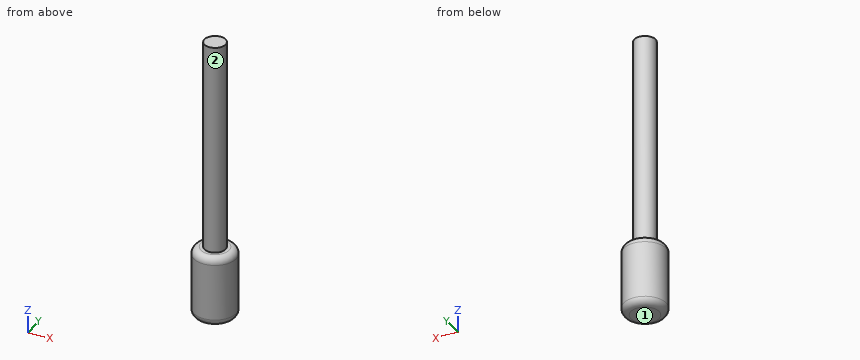
```python
from build123d import *

# Parameters (mm, degrees)
F0_R     = 15
F1_DEPTH = 50
F2_R     = 5
F3_R     = 7.5
F4_DEPTH = 150


with BuildPart() as f1:
    # F0 (on Top) → F1 (new body)
    with BuildSketch(Plane.XY):
        Circle(F0_R)
    extrude(amount=F1_DEPTH)

    # F2
    f2_edges = [f1.edges().sort_by_distance(p)[0] for p in [
        (-15, 0, 50),
        (-15, 0, 0),
    ]]
    fillet(f2_edges, radius=F2_R)

    # F3 (on face) → F4 (join)
    with BuildSketch(Plane.XY.offset(50)):
        Circle(F3_R)
    extrude(amount=F4_DEPTH)


solid = f1.part
```
Geometry: final body of the model. Coordinates: model frame, mm. Face numbers are marked on the shaded views. A direction names the side the tool comes from. Coordinates: 2 decimals unless noted, no trailing zeros. Order: outer loops, then holes, each group sorted by start corner. A loop starts at its lowest first (then second) coordinate and runs counter-clockwise, first axis right, second up. Notation, with made-up numbers: (47.5, 50.5) - (64.5, 50.5) arc R14 ccw to (64.5, 60.5) - close; hole circle Ø3 at (46, -29). An arc over 180 degrees is marked (long way). Write each question's results on one line, items separated by ' | '.
1) Set-up query: the marked faces 1 and 2. Return all of +Z, -Z, +X, -X, +Y, -Y with unobstructed straight access to the full face (end or side cutting, diameter ignored); none if empty.
Results list:
face 1: -Z, +X, -X, +Y, -Y | face 2: +Z
2) Pin query (flat end, axial travel): pin 1 (8 mm diameter, centred on x = 11.5, y = -11.5, fed in from -Z); pin 2 (6 mm diameter, centred on y = -5, z = 47.5, fed in from +X); pin 3 (1.5 mm diameter, centred on y = 9, z = 67.5, fed in from -X); pin 4 (2 mm diameter, centred on x = -2.5, z = 136, fed in from +Y). Return the tip coordinate at first contact, or that it passes through.
Results list:
pin 1: z = 0.54 | pin 2: x = 14.72 | pin 3: through | pin 4: y = 7.35
3) Section C-C, the plane z = 151.5. Return loops of the section in (x, y), plus the area to 3 significant figures.
Results list:
outline: circle Ø15 at (0, 0) | area: 177 mm^2
4) Section A-A, the plane y = 0. Return loops of the section in (x, z).
Results list:
outline: (-15, 5) arc R5 ccw to (-10, 0) - (10, 0) arc R5 ccw to (15, 5) - (15, 45) arc R5 ccw to (10, 50) - (7.5, 50) - (7.5, 200) - (-7.5, 200) - (-7.5, 50) - (-10, 50) arc R5 ccw to (-15, 45) - close
5) Line query: line 1 (Z direction, x = 2.5, y = -8); line 2 (Y direction, x = -1.5, z = 140.5); line 3 (X direction, y = 4, z = 180.5). Output: solid intervals per line, ascending. Write a range as from..to.
Results list:
line 1: 0..50 | line 2: -7.35..7.35 | line 3: -6.34..6.34
